Part print with two shaded views. Sizes in mm from the minimum x, y, z corner. Coordinates: 2 decimals unless noted, no trailing zeros. Loops run counter-clockwise (first coordinate to the right, second up) from the corner with the lowest first, then second, coordinate; pieces in that order, holes last.
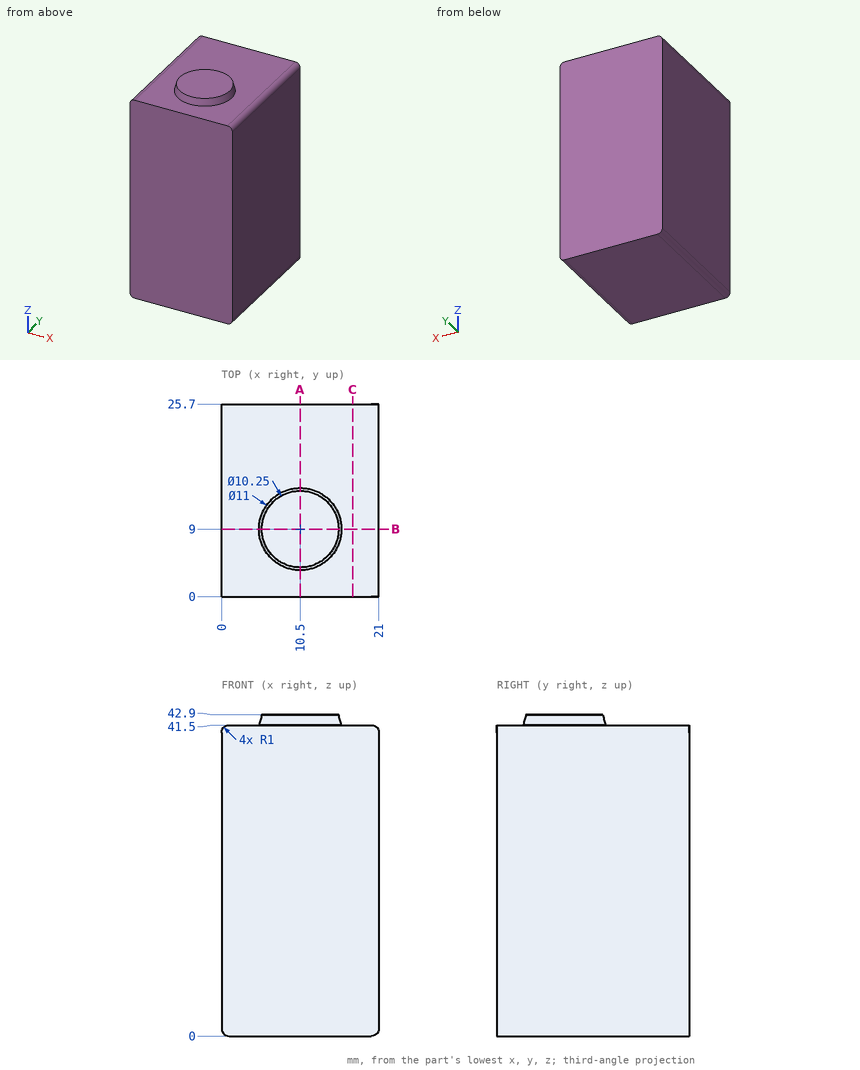
Q1. Slice it at B-B (y = 9). List the corners of the cut face in (x, z) (1 decimal).
Answers:
outline: (0, 1) arc R1 ccw to (1, 0) - (20, 0) arc R1 ccw to (21, 1) - (21, 40.5) arc R1 ccw to (20, 41.5) - (16, 41.5) - (15.6, 42.9) - (5.4, 42.9) - (5, 41.5) - (1, 41.5) arc R1 ccw to (0, 40.5) - close
Q2. Slice it at A-A (x = 10.5). List the corners of the cut face in (y, z) (1 decimal), and give its area (3 significant figures).
Answers:
outline: (0, 0) - (25.7, 0) - (25.7, 41.5) - (14.5, 41.5) - (14.1, 42.9) - (3.9, 42.9) - (3.5, 41.5) - (0, 41.5) - close
area: 1,080 mm2
Q3. Slice it at C-C (x = 17.5). List the corners of the cut face in (y, z).
Answers:
outline: (0, 0) - (25.7, 0) - (25.7, 41.5) - (0, 41.5) - close
Q4. Flat gauge pin, fed straight in: P1, Ø1.5, axis at x = 5, y = 17.5, coming from the +Z side. Where does the tip first touch, or does it go through?
Answers:
P1: stops at z = 41.5
Q5. Drill centre line: line 1 (Z direction, x = 17.75, y = 9.75). Where is it in solid material? Low to high.
Answers:
line 1: z = 0 to 41.5
